```python
from build123d import *

# Parameters (mm, degrees)
F0_W     = 3.175
F0_H     = 50.8
F0_H_2   = 22.225
F1_DEPTH = 22.225
F2_W     = 3.175
F2_H     = 76.2
F3_DEPTH = 25.4


# Not quite as in the source:
# - a feature names something its author has since deleted; it is built from what else it names


with BuildPart() as f1:
    # F0 (on Front) → F1 (new body, symmetric)
    with BuildSketch(Plane.XZ):
        Polygon((-3.175, 25.4), (0, 25.4), (9.525, 25.4), (12.7, 25.4), (19.4811138548, 25.4), (22.225, 25.4), (25.4, 25.4), (25.4, 28.575), (-25.4, 28.575), (-25.4, 25.4), (-22.225, 25.4), (-15.875, 25.4), (-12.7, 25.4), align=None)
        with Locations((-23.8125, 0)):
            Rectangle(F0_W, F0_H)
        with Locations((-14.2875, 0)):
            Rectangle(F0_W, F0_H)
        with Locations((23.8125, 0)):
            Rectangle(F0_W, F0_H)
        with Locations((11.1125, 0)):
            Rectangle(F0_W, F0_H)
        with Locations((-1.5875, 0)):
            Rectangle(F0_W, F0_H)
        Polygon((25.4, -25.4), (22.225, -25.4), (22.225, -47.625), (25.4, -47.625), (25.4, -39.3581977692), (25.4, -38.6990095903), (25.4, -31.6347628832), align=None)
        with Locations((-23.8125, -36.5125)):
            Rectangle(F0_W, F0_H_2)
    extrude(amount=F1_DEPTH, both=True)

    # F2 (on Right) → F3 (join, symmetric)
    with BuildSketch(Plane.YZ):
        with Locations((-23.8125, -9.525)):
            Rectangle(F2_W, F2_H)
        with Locations((23.8125, -9.525)):
            Rectangle(F2_W, F2_H)
    extrude(amount=F3_DEPTH, both=True)


solid = f1.part
```
Geometry: final body of the model. Coordinates: model frame, mm. A direction names the side the tool comes from. Coordinates: 2 decimals unless noted, no trailing zeros. Write each loop counter-clockwise with the first axis right and the second up, starting at its lowest first coordinate (ties: lowest second). Pieces come first, ordered by that corner, then holes. Notation, with made-up numbers: M -39.75,-39 L 19.25,-39 A22 cw 19.25,-15 Z; hole C 78,46 d11. An arc over 180 degrees is marked long. Use CSV: the item, a comma, the result in double quotes. Start each with the question number.
1. First-contact query: P1, Ø3, axis at x = 17, y = 8, coming from the -Z side; P2, Ø3.5, axis at x = -13.5, y = -9, coming from the -Z side. Flat tips, straight axial feed; report the tip coordinate or a pass-through.
2. Ray query, probe 1 along X at (y, z) = (15.5, -25) (3 decimals); probe 2 along Y at (x, z) = (-6, 23) (3 decimals). Return the intervals inside material, ascending.
3. Cut plane D-D on x = 3. Return the cut outline in (y, z) (3 decimals).
4. Cut plane B-B on z = -29. Return the cut outline in (x, y) (3 decimals), plus the area to 3 significant figures.
5. Mould query, pull axis Y, two halves, no side actions, for faces 1 (the face through (0, -25.4, -10)), 2 (the face through (5, 0, 25.4)), 3 (the face through (0, 25.4, -10)). Classes: pulls with the +Y half, pulls with the -Y half, needs draft (parallel to the pull), parting line crosses it, or undercut.
6. Cut plane A-A on z = 5. Return the cut outline in (x, y) (3 decimals).
7. Reachability of faces 4 (the face through (-25.4, 0, -9)), 5 (the face through (-14, 0, -25.4)) from +Z, -Z, +X, -X, +Y, -Y: full face, straight path, thin tool, end or side. Return the list, or none.
8. Cut plane C-C on y = -13.5. Return the cut outline in (x, z) (3 decimals).
Entries:
1,P1,"z = 25.4"
1,P2,"z = -25.4"
2,probe 1,"-25.4 to -22.225, -15.875 to -12.7, -3.175 to 0, 9.525 to 12.7, 22.225 to 25.4"
2,probe 2,"-25.4 to -22.225, 22.225 to 25.4"
3,outline,"M -25.4,-47.625 L -22.225,-47.625 L -22.225,25.4 L 22.225,25.4 L 22.225,-47.625 L 25.4,-47.625 L 25.4,28.575 L -25.4,28.575 Z"
4,outline,"M -25.4,-25.4 L 25.4,-25.4 L 25.4,25.4 L -25.4,25.4 Z; hole M -22.225,-22.225 L 22.225,-22.225 L 22.225,22.225 L -22.225,22.225 Z"
4,area,"605 mm²"
5,face 1,"pulls with the -Y half"
5,face 2,"undercut"
5,face 3,"pulls with the +Y half"
6,outline,"M -25.4,-25.4 L 25.4,-25.4 L 25.4,25.4 L -25.4,25.4 Z; hole M -22.225,-22.225 L -15.875,-22.225 L -15.875,22.225 L -22.225,22.225 Z; hole M -12.7,-22.225 L -3.175,-22.225 L -3.175,22.225 L -12.7,22.225 Z; hole M 0,-22.225 L 9.525,-22.225 L 9.525,22.225 L 0,22.225 Z; hole M 12.7,-22.225 L 22.225,-22.225 L 22.225,22.225 L 12.7,22.225 Z"
7,face 4,"+Z, -Z, -X, +Y, -Y"
7,face 5,"-Z"
8,outline,"M -25.4,-47.625 L -22.225,-47.625 L -22.225,25.4 L -15.875,25.4 L -15.875,-25.4 L -12.7,-25.4 L -12.7,25.4 L -3.175,25.4 L -3.175,-25.4 L 0,-25.4 L 0,25.4 L 9.525,25.4 L 9.525,-25.4 L 12.7,-25.4 L 12.7,25.4 L 22.225,25.4 L 22.225,-47.625 L 25.4,-47.625 L 25.4,28.575 L -25.4,28.575 Z"
